```python
from build123d import *

# Parameters (mm, degrees)
BOSS_EXTRUDE1_DEPTH = 44
CUT_EXTRUDE1_DEPTH  = 19
CUT_EXTRUDE2_DEPTH  = 22
CUT_EXTRUDE3_DEPTH  = 19
CUT_EXTRUDE4_DEPTH  = 19
CUT_EXTRUDE5_DEPTH  = 15
FILLET1_R           = 2
FILLET2_R           = 5


with BuildPart() as part:
    # Sketch1 → Boss-Extrude1 (new body)
    with BuildSketch(Plane(origin=(0, 0, 0), x_dir=(1, 0, 0), z_dir=(0, 1, 0))):
        with BuildLine():
            Line((33.8, 41.5), (0, 41.5))
            Line((0, 41.5), (0, 0))
            Line((0, 0), (41.5, 0))
            Line((41.5, 0), (41.5, 33.8))
            ThreePointArc((41.5, 33.8), (36.055277785, 36.055277785), (33.8, 41.5))
        make_face()
    extrude(amount=BOSS_EXTRUDE1_DEPTH)

    # Sketch2 → Cut-Extrude1 (cut)
    with BuildSketch(Plane(origin=(0, 44, 0), x_dir=(1, 0, 0), z_dir=(0, 1, 0))):
        Polygon((6.330417381, 0), (0, 0), (0, 4.89140223), (27.514137546, 40.5), (33.844554927, 35.60859777), align=None)
    extrude(amount=-CUT_EXTRUDE1_DEPTH, mode=Mode.SUBTRACT)

    # Sketch3 → Cut-Extrude2 (cut)
    with BuildSketch(Plane(origin=(0, 44, 0), x_dir=(1, 0, 0), z_dir=(0, 1, 0))):
        Polygon((6.165208691, 12.870370718), (23.285116497, 35.026831552), (20.119907806, 37.472532667), (3, 15.316071833), align=None)
    extrude(amount=-CUT_EXTRUDE2_DEPTH, mode=Mode.SUBTRACT)

    # Sketch5 → Cut-Extrude3 (cut)
    with BuildSketch(Plane(origin=(0, 44, 0), x_dir=(1, 0, 0), z_dir=(0, 1, 0))):
        Polygon((11.268941532, 6.39140223), (33.280251569, 34.878280446), (39.61066895, 29.986878216), (17.599358914, 1.5), align=None)
    extrude(amount=-CUT_EXTRUDE3_DEPTH, mode=Mode.SUBTRACT)

    # Sketch6 → Cut-Extrude4 (cut)
    with BuildSketch(Plane(origin=(0, 44, 0), x_dir=(1, 0, 0), z_dir=(0, 1, 0))):
        Polygon((17.599358914, 1.5), (16.440335282, 0), (0, 0), (0, 11.433493535), (3, 15.316071833), (6.165208691, 12.870370718), (11.268941532, 6.39140223), align=None)
    extrude(amount=-CUT_EXTRUDE4_DEPTH, mode=Mode.SUBTRACT)

    # Sketch7 → Cut-Extrude5 (cut)
    with BuildSketch(Plane(origin=(0, 44, 0), x_dir=(1, 0, 0), z_dir=(0, 1, 0))):
        Polygon((22.759033969, 0), (41.5, 24.254422662), (41.5, 0), align=None)
        Polygon((0, 19.611107666), (16.913162329, 41.5), (0, 41.5), align=None)
    extrude(amount=-CUT_EXTRUDE5_DEPTH, mode=Mode.SUBTRACT)

    # Fillet1
    # the kernel refuses this fillet: 2 mm, written as the material it takes off along each edge
    with BuildSketch(Plane(origin=(33.280251569, 48.213017341, -34.878280446), x_dir=(0.7913021726593984, 0, 0.6114252787908885), z_dir=(0, -1, 0))) as fillet1_piece_1:
        with BuildLine():
            CenterArc((1.685206936, -2), FILLET1_R, 90, 57.416069246)
            Line((0, -0.922931023), (0, 0))
            Line((0, 0), (1.685206936, 0))
        make_face()
    extrude(amount=23.213017341, mode=Mode.SUBTRACT)
    with BuildSketch(Plane(origin=(23.285116497, 49, -35.026831552), x_dir=(0.6114252787908897, 0, -0.7913021726593975), z_dir=(0, -1, 0))) as fillet1_piece_2:
        with BuildLine():
            CenterArc((FILLET1_R, -FILLET1_R), FILLET1_R, 90, 90)
            Line((0, -FILLET1_R), (0, 0))
            Line((0, 0), (FILLET1_R, 0))
        make_face()
    extrude(amount=24, mode=Mode.SUBTRACT)
    with BuildSketch(Plane(origin=(16.440335282, 54.182110795, 0), x_dir=(1, 0, 0), z_dir=(0, -1, 0))) as fillet1_piece_3:
        with BuildLine():
            CenterArc((FILLET1_R * 2.0364221589, -FILLET1_R), FILLET1_R, 90, 127.692631401)
            Line((FILLET1_R * 1.24511998624, -FILLET1_R * 1.61142527879), (0, 0))
            Line((0, 0), (FILLET1_R * 2.0364221589, 0))
        make_face()
    extrude(amount=29.182110795, mode=Mode.SUBTRACT)
    with BuildSketch(Plane(origin=(0, 58.64857796, -11.433493535), x_dir=(0, 0, -1), z_dir=(0, -1, 0))) as fillet1_piece_4:
        with BuildLine():
            CenterArc((FILLET1_R * 2.92971559207, FILLET1_R), FILLET1_R, 127.692631401, 142.307368599)
            Line((FILLET1_R * 2.31829031328, FILLET1_R * 1.79130217266), (0, 0))
            Line((0, 0), (FILLET1_R * 2.92971559207, 0))
        make_face()
    extrude(amount=33.64857796, mode=Mode.SUBTRACT)
    with BuildSketch(Plane(origin=(0, 58.64857796, -11.433493535), x_dir=(0, 0, -1), z_dir=(0, -1, 0))) as fillet1_piece_5_section:
        with BuildLine():
            CenterArc((FILLET1_R * 2.92971559207, FILLET1_R), FILLET1_R, 127.692631401, 142.307368599)
            Line((FILLET1_R * 2.31829031328, FILLET1_R * 1.79130217266), (0, 0))
            Line((0, 0), (FILLET1_R * 2.92971559207, 0))
        make_face()
    fillet1_piece_5 = extrude(amount=48.297155921, mode=Mode.PRIVATE)
    fillet1_piece_5 = split(fillet1_piece_5, bisect_by=Plane(origin=(2.943298817, 23.5, -15.35988384), z_dir=(0.6114252787908899, 0, -0.7913021726593973)), keep=Keep.TOP, mode=Mode.PRIVATE)
    fillet1_piece_5 = split(fillet1_piece_5, bisect_by=Plane(origin=(3.087132223, 22, -15.546031994), z_dir=(0, 1, 0)), keep=Keep.TOP, mode=Mode.PRIVATE)
    add(fillet1_piece_5, mode=Mode.SUBTRACT)

    # Fillet2
    fillet2_edges = [part.edges().sort_by_distance(p)[0] for p in [
        (32.129516985, 29, -12.127211331),
        (8.456581164, 29, -30.555553833),
    ]]
    fillet(fillet2_edges, radius=FILLET2_R)


solid = part.part
```
Geometry check sheet. Reference: the model listing, model coordinates, mm. A direction names the side the tool comes from. Coordinates: 2 decimals unless noted, no trailing zeros. Order: outer loops, then holes, each group sorted by start corner. A loop starts at its lowest first (then second) coordinate and runs counter-clockwise, first axis right, second up. Notation, with made-up numbers: (-23, 4.25) - (26, 4.25) arc R28 cw to (26, 25.25) - close; hole circle Ø11 at (84, -6.5). An arc over 180 degrees is marked (long way). Answer in a Markdown table with one row per item. Add a question column.
1. Section check C-C (y = 30). Enter the section's corners in (x, z), plus the area to 3 significant figures.
2. Access from +Z, -Z, +X, -X, +Y, -Y to the whole of each face (thin tool, end or side, straight path). Record for faces 5 (the face through (18.73, 34.63, -1.09)), 6 (the face through (17, 17, -41.5)), 7 (the face through (29.415, 34.633, -16.792)).
3. Gauge pin test, flat ends, axial feed: pin 1 Ø3 at (x, z) = (6, -31) entering from +Y; pin 2 Ø8 at (x, z) = (7.5, -34) entering from +Y; pin 3 Ø12 at (x, z) = (26.5, -24.5) entering from +Y; pin 4 Ø10 at (x, z) = (37, -9.5) entering from +Y. Record the tip position at first contact, or that the pin passes through.
4. Section check B-B (y = 36). Enter the section's corners in (x, z), plus the area to 3 significant figures.
5. Draft check along Z on faces 1 (the face through (33.5, 30.4, -11.4)), 2 (the face through (23.2, 34.63, -35.85)), 3 (the face through (0, 12, -21)), 4 (the face through (36.115, 21.692, -35.996)). Enter one of: +Z half, -Z half, draft (parallel to the pull), parting line (faces both ways), or undercut.
6. Section check A-A (y = 10). Enter the section's corners in (x, z).
7. Material ranges on L1, parallel to Y at x = 26.5, z = -38.5; L2, parallel to Z at x = 19, y = 33.5; L3, parallel to X at y = 41.5, z = -20, recorded low to high. Write a range as [from, to].
Data:
| question | item | result |
|---|---|---|
| 1 | outline | (0, -22.88) - (14.39, -41.5) - (33.8, -41.5) arc R7.7 cw to (41.5, -33.8) - (41.5, -20.98) - (25.29, 0) - (20.51, 0) arc R2 ccw to (18.93, -3.22) - (39.61, -29.99) - (34.61, -33.85) arc R2 ccw to (33.84, -35.61) - (27.51, -40.5) - (24.51, -36.61) arc R2 ccw to (21.7, -36.25) - (20.12, -37.47) - (3.58, -16.07) arc R2 ccw to (0, -17.29) - close |
| 1 | area | 515 mm² |
| 2 | face 5 | -X, +Y |
| 2 | face 6 | -Z, +X, -X, +Y, -Y |
| 2 | face 7 | +Y |
| 3 | pin 1 | stops at y = 31.42 |
| 3 | pin 2 | stops at y = 44 |
| 3 | pin 3 | stops at y = 25 |
| 3 | pin 4 | stops at y = 31.9 |
| 4 | outline | (0, -19.61) - (16.91, -41.5) - (33.8, -41.5) arc R7.7 cw to (41.5, -33.8) - (41.5, -24.25) - (22.76, 0) - (20.51, 0) arc R2 ccw to (18.93, -3.22) - (39.61, -29.99) - (34.61, -33.85) arc R2 ccw to (33.84, -35.61) - (27.51, -40.5) - (24.51, -36.61) arc R2 ccw to (21.7, -36.25) - (20.12, -37.47) - (3.58, -16.07) arc R2 ccw to (0, -17.29) - close |
| 4 | area | 406 mm² |
| 5 | face 1 | +Z half |
| 5 | face 2 | undercut |
| 5 | face 3 | draft |
| 5 | face 4 | -Z half |
| 6 | outline | (0, -41.5) - (33.8, -41.5) arc R7.7 cw to (41.5, -33.8) - (41.5, 0) - (0, 0) - close |
| 7 | L1 | y = [0, 25] |
| 7 | L2 | z = [-41.5, -36.02], [-3.31, -0.69] |
| 7 | L3 | x = [0.3, 6.62], [31.89, 38.21] |
